Geometry: final body of the model. Coordinates: model frame, mm. Face numbers are marked on the shaded views. Give positions to 0.01 mm unless a question says otherwise; leave off trailing zeros. Order: outer loops, then holes, each group sorted by start corner. A loop starts at its lowest first (then second) coordinate and runs counter-clockwise, first axis right, second up. Notation, with made-up numbers: (5.25, 34) - (34.25, 34) arc R16 ccw to (34.25, 43) - close; hole circle Ø6 at (-32.5, -24). An arc over 180 degrees is marked (long way). Use one line per item in the form item = value.
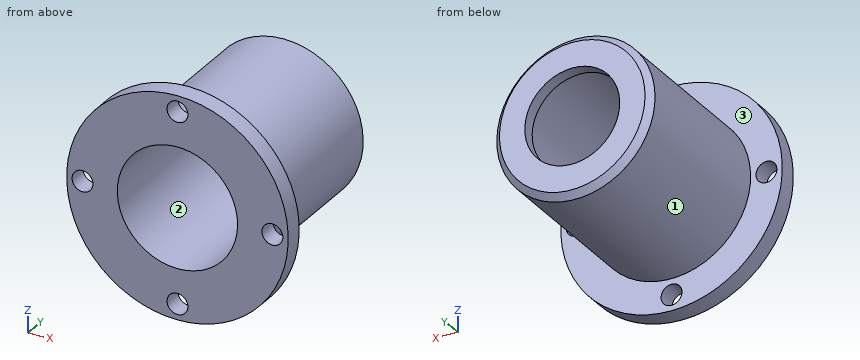
from build123d import *

# Parameters (mm, degrees)
SKETCH_1_R          = 17.5
EXTRUDE_1_DEPTH     = 3
SKETCH_2_R          = 12.5
EXTRUDE_2_DEPTH     = 27
SKETCH_4_R          = 9.5
CUT_EXTRUDE_1_DEPTH = 28
SKETCH_5_R          = 7.5
CUT_EXTRUDE_2_DEPTH = 28
CHAMFER_1_SIZE      = 1
SKETCH_6_R          = 1.65
CUT_EXTRUDE_3_DEPTH = 10


with BuildPart() as part:
    # Эскиз1 → Бобышка-Вытянуть1 (new body)
    with BuildSketch(Plane(origin=(0, 0, 0), x_dir=(1, 0, 0), z_dir=(0, 1, 0))):
        with Locations(Location((0, 0, 0), (0, 0, 270))):
            Circle(SKETCH_1_R)
    extrude(amount=EXTRUDE_1_DEPTH)

    # Эскиз2 → Бобышка-Вытянуть2 (add)
    with BuildSketch(Plane(origin=(0, 3, 0), x_dir=(1, 0, 0), z_dir=(0, 1, 0))):
        with Locations(Location((0, 0, 0), (0, 0, 270))):
            Circle(SKETCH_2_R)
    extrude(amount=EXTRUDE_2_DEPTH)

    # Эскиз4 → Вырез-Вытянуть1 (cut)
    with BuildSketch(Plane.XZ):
        with Locations(Location((0, 0, 0), (0, 0, 270))):
            Circle(SKETCH_4_R)
    extrude(amount=-CUT_EXTRUDE_1_DEPTH, mode=Mode.SUBTRACT)

    # Эскиз5 → Вырез-Вытянуть2 (cut)
    with BuildSketch(Plane(origin=(0, 30, 0), x_dir=(1, 0, 0), z_dir=(0, 1, 0))):
        with Locations(Location((0, 0, 0), (0, 0, 270))):
            Circle(SKETCH_5_R)
    extrude(amount=-CUT_EXTRUDE_2_DEPTH, mode=Mode.SUBTRACT)

    # Фаска1
    chamfer_1_edges = [part.edges().sort_by_distance(p)[0] for p in [
        (0, 30, -12.5),
    ]]
    chamfer(chamfer_1_edges, length=CHAMFER_1_SIZE)

    # Эскиз6 → Вырез-Вытянуть3 (cut)
    with BuildSketch(Plane.XZ):
        with Locations(Location((0, 15, 0), (0, 0, 270))):
            Circle(SKETCH_6_R)
        with Locations(Location((-15, 0, 0), (0, 0, 270))):
            Circle(SKETCH_6_R)
        with Locations(Location((0, -15, 0), (0, 0, 270))):
            Circle(SKETCH_6_R)
        with Locations(Location((15, 0, 0), (0, 0, 270))):
            Circle(SKETCH_6_R)
    extrude(amount=-CUT_EXTRUDE_3_DEPTH, mode=Mode.SUBTRACT)


solid = part.part
(1) Cut plane C-C on x = -15. Output: boundary loops of the cut face in (y, z).
Computed values:
outline = (0, -9.01) - (3, -9.01) - (3, -1.65) - (0, -1.65) - close; (0, 1.65) - (3, 1.65) - (3, 9.01) - (0, 9.01) - close
(2) Cut plane B-B on z = 0. Output: boundary loops of the cut face in (x, y).
Computed values:
outline = (-17.5, 0) - (-16.65, 0) - (-16.65, 3) - (-17.5, 3) - close; (-13.35, 0) - (-9.5, 0) - (-9.5, 28) - (-7.5, 28) - (-7.5, 30) - (-11.5, 30) - (-12.5, 29) - (-12.5, 3) - (-13.35, 3) - close; (7.5, 28) - (9.5, 28) - (9.5, 0) - (13.35, 0) - (13.35, 3) - (12.5, 3) - (12.5, 29) - (11.5, 30) - (7.5, 30) - close; (16.65, 0) - (17.5, 0) - (17.5, 3) - (16.65, 3) - close
(3) Cut plane D-D on z = -15. Output: boundary loops of the cut face in (x, y), plus the area to 3 significant figures.
Computed values:
outline = (-9.01, 0) - (-1.65, 0) - (-1.65, 3) - (-9.01, 3) - close; (1.65, 0) - (9.01, 0) - (9.01, 3) - (1.65, 3) - close
area = 44.2 mm²
(4) Pull-direction query (X, two-part tool) for the marked faces 1, 2 and 3; classes: released by +X, released by -X, zero draft, split by the parting line, or undercut.
Computed values:
face_1 = split by the parting line
face_2 = undercut
face_3 = zero draft
(5) Cut plane A-A on x = 0. Output: boundary loops of the cut face in (y, z).
Computed values:
outline = (0, -17.5) - (3, -17.5) - (3, -16.65) - (0, -16.65) - close; (0, -13.35) - (3, -13.35) - (3, -12.5) - (29, -12.5) - (30, -11.5) - (30, -7.5) - (28, -7.5) - (28, -9.5) - (0, -9.5) - close; (0, 9.5) - (28, 9.5) - (28, 7.5) - (30, 7.5) - (30, 11.5) - (29, 12.5) - (3, 12.5) - (3, 13.35) - (0, 13.35) - close; (0, 16.65) - (3, 16.65) - (3, 17.5) - (0, 17.5) - close
(6) Ray query, line 1 along X through (y, z) = (8, 0); line 2 along Y through (x, z) = (-8.5, 3.5); line 3 along Z through (x, y) = (-5.5, 2). Return the intervals inside material, ascending.
Computed values:
line_1 = -12.5 to -9.5, 9.5 to 12.5
line_2 = 28 to 30
line_3 = -16.61 to -7.75, 7.75 to 16.61
(7) Contact query for flat-ended pins moving along their axis: pin 1 Ø5 at (y, z) = (15, 11.5) entering from +X; pin 2 Ø2 at (x, y) = (-11, 7) entering from +Z; pin 3 Ø10 at (y, z) = (7.5, -12) entering from -X. Output: stop coordinate, or through.
Computed values:
pin_1 = 8.67
pin_2 = 7.5
pin_3 = -14.48
